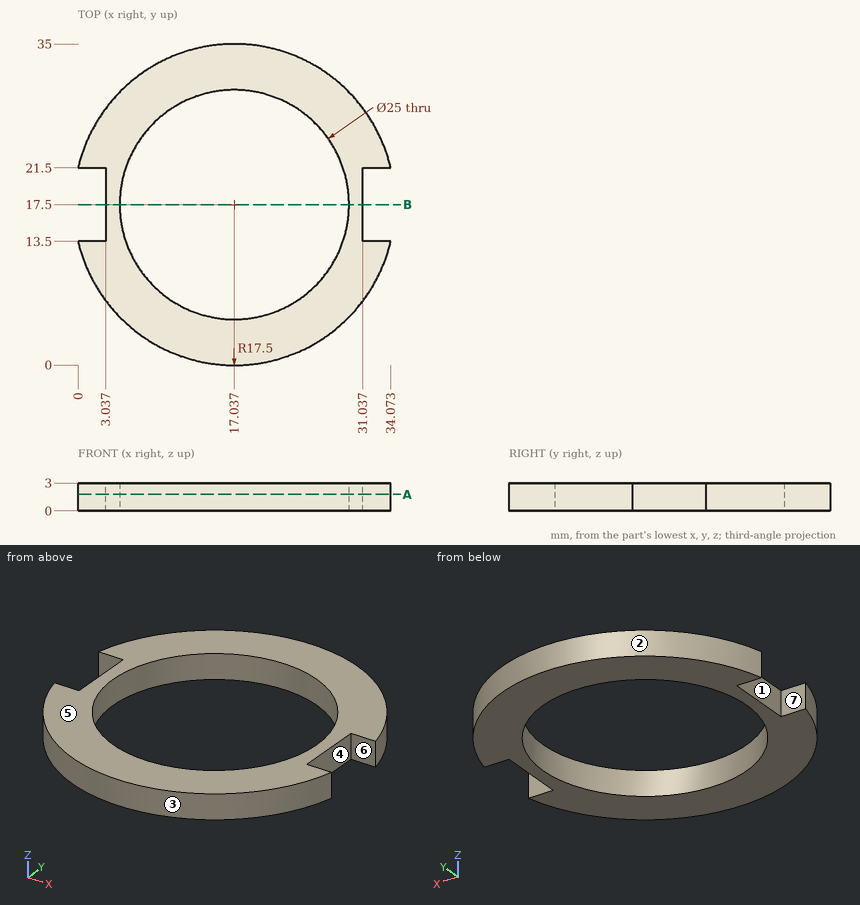
Can you work these out from the drawing? Everything is in mm from the part's minimum corner. A direction names the side the tool comes from. Coordinates: 2 decimals unless noted, no trailing zeros. Loops run counter-clockwise (first coordinate to the right, second up) from the corner with the lowest first, then second, coordinate; pieces in that order, holes last.
1) Will these pins go through, and if not, where does the flat tip stop? pin 1 Ø1 at (y, z) = (12, 2.5) entering from -X; pin 2 Ø1.5 at (y, z) = (5.5, 2.5) entering from -X; pin 3 Ø1.5 at (x, z) = (33, 1) entering from +Y.
Reported:
pin 1: stops at x = 0.27
pin 2: stops at x = 3.63
pin 3: stops at y = 26.15
2) Thinking about a two-plate mould opening in Y: for the marked faces 1, 2, 3 and 4, which applies, released by +Y, released by -Y, zero draft, split by the parting line, or undercut?
Reported:
face 1: undercut
face 2: released by +Y
face 3: released by -Y
face 4: undercut
3) Which directions (+Z, -Z, +X, -X, +Y, -Y) give clear straight access to the entire face, cutting with the end or side of a thin tool? Please do the marked faces 5, 6 and 7.
Reported:
face 5: +Z, +X, -X, +Y, -Y
face 6: +Z, -Z, +X
face 7: +Z, -Z, -X
4) Please list where these lines run through material, in increasing order: line 1 along X through (y, z) = (18, 2.85); line 2 along Y through (x, z) = (3, 2.6); line 3 along Y through (x, z) = (9.5, 1.5) (1 decimal).
Reported:
line 1: x = 3.04 to 4.55, 29.53 to 31.04
line 2: y = 7.05 to 13.5, 21.5 to 27.95
line 3: y = 1.7 to 7.5, 27.5 to 33.3
5) Imagine slicing it at B-B (y = 17.5). List the corners of the cut face in (x, z) for me.
Reported:
outline: (3.04, 0) - (4.54, 0) - (4.54, 3) - (3.04, 3) - close; (29.54, 0) - (31.04, 0) - (31.04, 3) - (29.54, 3) - close
6) Imagine slicing it at A-A (z = 1.8). List the corners of the cut face in (x, y) for me.
Reported:
outline: (0, 13.5) arc R17.5 ccw to (34.07, 13.5) - (31.04, 13.5) - (31.04, 21.5) - (34.07, 21.5) arc R17.5 ccw to (0, 21.5) - (3.04, 21.5) - (3.04, 13.5) - close; hole circle Ø25 at (17.04, 17.5)
